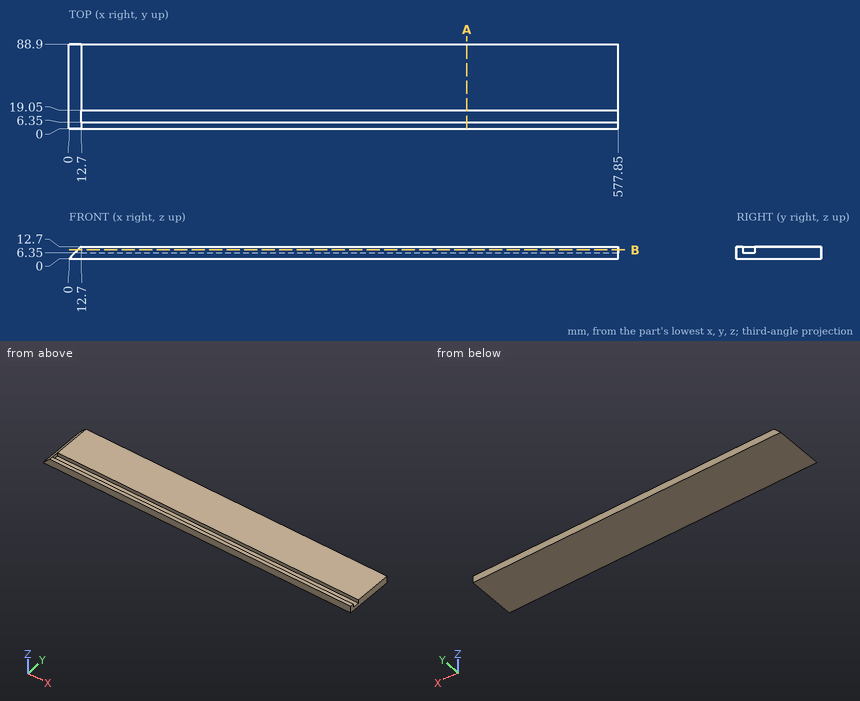
Answer from the drawing. Dimensions are ordinates in mm from the lowest x, y and z of the part. Coordinates: 2 decimals unless noted, no trailing zeros. Loops run counter-clockwise (first coordinate to the right, second up) from the corner with the lowest first, then second, coordinate; pieces in that order, holes last.
1) Flat-ended cylindrical pins translate along their axes: pin 1 (3 mm diameter, centred on y = 12.5, z = 8, fed in from +X); pin 2 (3 mm diameter, centred on y = 40, z = 8.5, fed in from -X). Find the tip coordinate at first contact, or state that the pin passes through.
Results:
pin 1: stops at x = 12.7
pin 2: stops at x = 7
2) Consider probe 1 along Y at (x, z) = (496, 6.75); probe 2 along X at (y, z) = (13, 6.25); probe 3 along Z at (x, y) = (501, 7.5). Determine where each line is inside the solid, lowest interval first.
Results:
probe 1: y = 0 to 6.35, 19.05 to 88.9
probe 2: x = 6.25 to 577.85
probe 3: z = 0 to 6.35
3) Section A-A (x = 418.5) is taken. Give the vertices of the cut face in (y, z).
Results:
outline: (0, 0) - (88.9, 0) - (88.9, 12.7) - (19.05, 12.7) - (19.05, 6.35) - (6.35, 6.35) - (6.35, 12.7) - (0, 12.7) - close
4) Section B-B (z = 9.25) is taken. Give the vertices of the cut face in (x, y).
Results:
outline: (9.25, 0) - (577.85, 0) - (577.85, 6.35) - (12.7, 6.35) - (12.7, 19.05) - (577.85, 19.05) - (577.85, 88.9) - (9.25, 88.9) - close
